Here's how the part is built. I have some questions about the finished solid (model axes, mm). Face numbers are marked on the shaded views. A direction names the side the tool comes from. Give positions to 0.01 mm unless a question says otherwise; leave off trailing zeros. Loops run counter-clockwise (first coordinate to the right, second up) from the corner with the lowest first, then second, coordinate; pieces in that order, holes last.
Q1. I need wall thicknesses on probe 1 along Z at (x, y) = (-11, -12.7); probe 2 along X at (y, z) = (-13.75, 63); probe 3 along X at (y, z) = (-13.8, 119.5). Which ranges of each line are inside material? Lowest first, please.
Q2. Suppose I cut it at A-A (x = -16). List the corners of the cut face in (y, z) for me, and give its area (3 significant figures).
Q3. I'm going to push flat-ended pins straight in: P1, Ø11, axis at x = -6.5, z = 39.5, coming from the +Y side; P2, Ø6, axis at y = -8, z = 73, coming from the -X side; P3, Ø3.5, axis at y = -6, z = 37.5, coming from the -X side. Where does each tip first touch, or does it pass through?
Q4. For the marked faces 1 and 2, which set-ups out of +Z, -Z, +X, -X, +Y, -Y let a thin tool reach every point of the face, with its end or its side?
Q5. Suppose I cut it at C-C (x = -11). List the corners of the cut face in (y, z) for me.
Q6. Suppose I cut it at D-D (z = 50.5). List the corners of the cut face in (x, y) for me.
Q7. Suppose I cut it at B-B (z = 101). List the corners of the cut face in (x, y) for me.
```python
from build123d import *

# Parameters (mm, degrees)
SALIENTE_EXTRUIR1_DEPTH = 126
CROQUIS2_R              = 3
CORTAR_EXTRUIR3_DEPTH   = 63
CROQUIS3_R              = 3
CROQUIS3_R_2            = 3.243437353
CROQUIS3_R_3            = 3.351130608
CORTAR_EXTRUIR4_DEPTH   = 10


with BuildPart() as part:
    # Croquis1 → Saliente-Extruir1 (new body)
    with BuildSketch(Plane.XY):
        Polygon((0, 0), (3, 0), (3, -15), (-22, -15), (-22, -12), (0, -12), align=None)
    extrude(amount=SALIENTE_EXTRUIR1_DEPTH)

    # Croquis2 → Cortar-Extruir3 (cut, symmetric)
    with BuildSketch(Plane(origin=(3, 0, 0), x_dir=(0, 0, -1), z_dir=(1, 0, 0))):
        with Locations((-113.5, -6)):
            Circle(CROQUIS2_R)
        with Locations((-101, -6)):
            Circle(CROQUIS2_R)
        with Locations((-88.5, -6)):
            Circle(CROQUIS2_R)
        with Locations((-12.5, -6)):
            Circle(CROQUIS2_R)
        with Locations((-25, -6)):
            Circle(CROQUIS2_R)
        with Locations((-37.5, -6)):
            Circle(CROQUIS2_R)
    extrude(amount=CORTAR_EXTRUIR3_DEPTH, both=True, mode=Mode.SUBTRACT)

    # Croquis3 → Cortar-Extruir4 (cut)
    with BuildSketch(Plane(origin=(0, -12, 0), x_dir=(1, 0, 0), z_dir=(0, 1, 0))):
        with Locations((-11, -6.5)):
            Circle(CROQUIS3_R)
        with Locations((-11, -119.5)):
            Circle(CROQUIS3_R)
        with Locations((-16, -63)):
            Circle(CROQUIS3_R_2)
        with Locations((-6, -63)):
            Circle(CROQUIS3_R_3)
    extrude(amount=-CORTAR_EXTRUIR4_DEPTH, mode=Mode.SUBTRACT)


solid = part.part
```
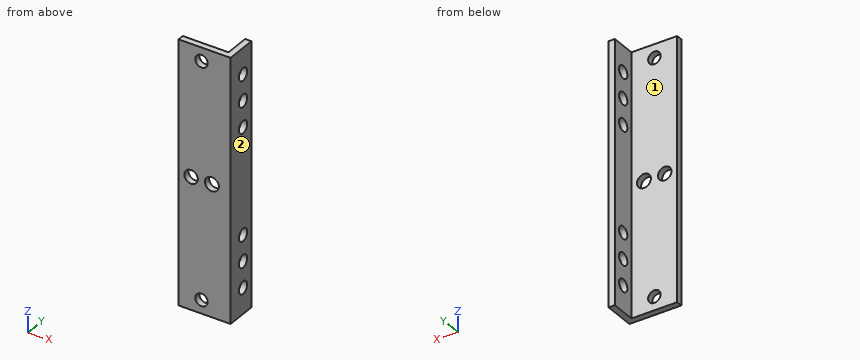
Solutions:
1. probe 1: z = 0 to 3.5, 9.5 to 116.5, 122.5 to 126
1. probe 2: x = -22 to -19.24, -12.76 to -9.35, -2.65 to 3
1. probe 3: x = -22 to -14, -8 to 3
2. outline: (-15, 0) - (-12, 0) - (-12, 59.76) - (-15, 59.76) - close; (-15, 66.24) - (-12, 66.24) - (-12, 126) - (-15, 126) - close
2. area: 359 mm2
3. P1: stops at y = -12
3. P2: stops at x = 0
3. P3: passes through
4. face 1: +Z, -Z, -X, +Y
4. face 2: +Z, -Z, +X, +Y, -Y
5. outline: (-15, 0) - (-12, 0) - (-12, 3.5) - (-15, 3.5) - close; (-15, 9.5) - (-12, 9.5) - (-12, 116.5) - (-15, 116.5) - close; (-15, 122.5) - (-12, 122.5) - (-12, 126) - (-15, 126) - close
6. outline: (-22, -15) - (3, -15) - (3, 0) - (0, 0) - (0, -12) - (-22, -12) - close
7. outline: (-22, -15) - (3, -15) - (3, -9) - (0, -9) - (0, -12) - (-22, -12) - close; (0, -3) - (3, -3) - (3, 0) - (0, 0) - close
